Geometry: final body of the model. Coordinates: model frame, mm. A direction names the side the tool comes from. Give positions to 0.01 mm unless a question says otherwise; leave off trailing zeros. Write each loop counter-clockwise with the first axis right and the second up, starting at its lowest first coordinate (ties: lowest second). Pieces come first, ordered by that corner, then holes. Notation, with made-up numbers: (42, 15) -> (69, 15) arc R15 cw to (69, 37) -> close; hole circle Ø3 at (-19.5, 81.5). An arc over 180 degrees is marked (long way). Answer as a JSON object with one key per item and string values.
from build123d import *

# Parameters (mm, degrees)
SKETCH009_R      = 1.8
EXTRUDE008_DEPTH = 5
SKETCH008_R      = 2.1
EXTRUDE007_DEPTH = 5


with BuildPart() as extrude008:
    # Sketch009 → Extrude008 (new body)
    with BuildSketch(Plane.XY):
        with BuildLine():
            Line((-21.002502, -42), (21.002502, -42))
            ThreePointArc((23, -44.1), (22.451639, -42.621595), (21.002502, -42))
            Line((23, -47.1), (23, -44.1))
            ThreePointArc((21, -49.1), (22.414214, -48.514214), (23, -47.1))
            Line((21, -49.1), (-21, -49.1))
            ThreePointArc((-23, -47.1), (-22.414214, -48.514214), (-21, -49.1))
            Line((-23, -47.1), (-23, -44.1))
            ThreePointArc((-21.002502, -42), (-22.451639, -42.621595), (-23, -44.1))
        make_face()
        with Locations((-18, -45)):
            Circle(SKETCH009_R, mode=Mode.SUBTRACT)
        with Locations((18, -45)):
            Circle(SKETCH009_R, mode=Mode.SUBTRACT)
    extrude(amount=EXTRUDE008_DEPTH)


with BuildPart() as extrude008_1:
    # Extrude008 placement: moved
    add(extrude008.part.moved(Location((0, 0, 11.2))))


with BuildPart() as obj1:
    # Sketch008 → Extrude007 (new body)
    with BuildSketch(Plane.YZ):
        with BuildLine():
            Line((-49, 11.2), (-40, 11.2))
            Line((-40, 11.2), (-22.745353, 8.64111))
            ThreePointArc((-22.745353, 8.64111), (-18.398196, 12.120519), (-22.187904, 16.2))
            Line((-22.187904, 16.2), (-49, 16.2))
            Line((-49, 16.2), (-49, 11.2))
        make_face()
        with Locations((-22.187904, 12.4)):
            Circle(SKETCH008_R, mode=Mode.SUBTRACT)
    extrude(amount=EXTRUDE007_DEPTH)


with BuildPart() as obj1_1:
    # Extrude007 placement: moved
    add(obj1.part.moved(Location((4, 0, 0))))

    # Fusion009: union Extrude008
    add(extrude008_1.part)


solid = obj1_1.part
Q1. First-contact query: P1, Ø3, axis at y = -34, z = 14, coming from the -X side; P2, Ø10, axis at x = -8.5, y = -33, coming from the +Z side; P3, Ø5, axis at x = 6.5, y = -28.5, coming from the -Z side; P4, Ø2.5, axis at x = -7, z = 13, coming from the +Y side. Flat tips, straight axial feed; report the tip coordinate or a pass-through.
Values:
{"P1": "x = 4", "P2": "through", "P3": "z = 9.12", "P4": "y = -42"}
Q2. Mould query, pull axis X, two halves, no side actions, for faces 1 (the cylindrical face through (22.47, -42.64, 13.66)), 2 (the cylindrical face through (-18.234, -43.215, 13.665)), 3 (the cylindrical face through (17.766, -43.215, 13.665)), 4 (the flat face through (4, -30, 13)). Classes: pulls with the +X half, pulls with the -X half, needs draft (parallel to the pull), parting line crosses it, or undercut.
Values:
{"face 1": "pulls with the +X half", "face 2": "undercut", "face 3": "undercut", "face 4": "pulls with the -X half"}
Q3. Cut plane B-B (z = 12.4). Return the cut outline in (x, y), and give its area (3 significant figures).
Values:
{"outline": "(-23, -47.1) arc R2 ccw to (-21, -49.1) -> (21, -49.1) arc R2 ccw to (23, -47.1) -> (23, -44.1) arc R2 ccw to (21, -42) -> (9, -42) -> (9, -24.29) -> (4, -24.29) -> (4, -42) -> (-21, -42) arc R2 ccw to (-23, -44.1) -> close; (4, -20.09) -> (9, -20.09) -> (9, -18.39) -> (4, -18.39) -> close; hole circle Ø3.6 at (-18, -45); hole circle Ø3.6 at (18, -45)", "area": "400 mm²"}
Q4. Cut plane D-D (z = 15). Return the cut outline in (x, y).
Values:
{"outline": "(-23, -47.1) arc R2 ccw to (-21, -49.1) -> (21, -49.1) arc R2 ccw to (23, -47.1) -> (23, -44.1) arc R2 ccw to (21, -42) -> (9, -42) -> (9, -19.42) -> (4, -19.42) -> (4, -42) -> (-21, -42) arc R2 ccw to (-23, -44.1) -> close; hole circle Ø3.6 at (-18, -45); hole circle Ø3.6 at (18, -45)"}
Q5. Set-up query: faces 5 (the flat face through (-9, -42, 14)), 6 (the flat face through (9, -30, 13)), 7 (the flat face through (0, -45, 11.2)). Return all of +Z, -Z, +X, -X, +Y, -Y with unobstructed straight access to the full face (end or side cutting, diameter ignored); none if empty.
Values:
{"face 5": "+Z, -Z, -X, +Y", "face 6": "+Z, -Z, +X, +Y", "face 7": "-Z, +X, -X, -Y"}
Q6. Cut plane A-A (y = -45). Return the cut outline in (x, z).
Values:
{"outline": "(-23, 11.2) -> (-19.8, 11.2) -> (-19.8, 16.2) -> (-23, 16.2) -> close; (-16.2, 11.2) -> (16.2, 11.2) -> (16.2, 16.2) -> (-16.2, 16.2) -> close; (19.8, 11.2) -> (23, 11.2) -> (23, 16.2) -> (19.8, 16.2) -> close"}
Q7. Material intervals for L1, parallel to Y at x = -18, z = 12.35; L2, parallel to Y at x = 20, z = 12.5; L3, parallel to X at y = -39, z = 15, sorted ascending. Write a range as from..to.
Values:
{"L1": "-49.1..-46.8, -43.2..-42", "L2": "-49.1..-42", "L3": "4..9"}
Q8. Cut plane C-C (x = -18). Return the cut outline in (y, z), and give its area (3 significant figures).
Values:
{"outline": "(-49.1, 11.2) -> (-46.8, 11.2) -> (-46.8, 16.2) -> (-49.1, 16.2) -> close; (-43.2, 11.2) -> (-42, 11.2) -> (-42, 16.2) -> (-43.2, 16.2) -> close", "area": "17.5 mm²"}
